Design review of the part built by this model. Coordinates are the model's own, in mm. A direction names the side the tool comes from. Round coordinates to 2 decimals unless told otherwise and drop trailing zeros. Loops run counter-clockwise (first coordinate to the right, second up) from the corner with the lowest first, then second, coordinate; pieces in that order, holes last. Notation, with made-up numbers: (-39, 60.25) - (4, 60.25) arc R20 ccw to (4, 66.25) - close; hole circle Ø3 at (-31.5, -8). An arc over 180 degrees is marked (long way). Use one line per item in the form item = value. Start each with the question number.
(1) We need section A-A, the plane z = 17. Write out the cut boundary in (x, y), then the cut area to 3 significant figures.
(2) Machinability: for faces 1 (the cylindrical face through (998.479, 10.525, -90.019)), 2 (the cylindrical face through (991.297, 90.986, 1.4)), which of the approach directions +Z, -Z, +X, -X, +Y, -Y give a long, thin tool a straight path to every point of the face, cutting with its end or side? Answer none if there is none.
(3) The part is to be moulded in two halves that separate along Y. For faces 3 (the cylindrical face through (1.479, 9.981, -89.475)), 4 (the cylindrical face through (2, 34, -52)), 5 (the flat face through (3, 39, 0)), say which applies: released by +Y, released by -Y, zero draft, split by the parting line, or undercut.
(4) Wall thickness on probe 1 along X at (y, z) = (57, -40.5); probe 2 along Y at (x, z) = (798.5, 64.5); probe 3 along X at (y, z) = (95.5, -28.5): over which ranges is each line inside the solid? List them lowest first. Write a range as [from, to].
(5) We need section B-B, the plane x = 613.5. Write out the cut boundary in (y, z), then the cut area to 3 significant figures.
(6) For pin 1 (1.5 mm diameter, centred on y = 89.5, z = -57, fed in from +X); pin 2 (8 mm diameter, centred on x = 395.5, z = 67.5, fed in from -Y), all flat-tipped, find the tip position at first contact; note any pin that passes through.
(7) We need section C-C, the plane z = 74.5. Write out the cut boundary in (x, y).
from build123d import *

# Parameters (mm, degrees)
BOSS_EXTRUDE1_DEPTH = 100
CUT_EXTRUDE1_DEPTH  = 1001
SKETCH4_R           = 10
CUT_EXTRUDE2_DEPTH  = 1001
FILLET3_R           = 35


with BuildPart() as part:
    # Sketch2 → Boss-Extrude1 (new body, symmetric)
    with BuildSketch(Plane.XY):
        with BuildLine():
            Line((0, 0), (0, 80))
            ThreePointArc((0, 80), (5.857864376, 94.142135624), (20, 100))
            Line((20, 100), (980, 100))
            ThreePointArc((980, 100), (994.142135624, 94.142135624), (1000, 80))
            Line((1000, 80), (1000, 0))
            Line((1000, 0), (997, 0))
            Line((997, 0), (997, 77))
            ThreePointArc((997, 77), (991.142135624, 91.142135624), (977, 97))
            Line((977, 97), (23, 97))
            ThreePointArc((23, 97), (8.857864376, 91.142135624), (3, 77))
            Line((3, 77), (3, 0))
            Line((3, 0), (0, 0))
        make_face()
    extrude(amount=BOSS_EXTRUDE1_DEPTH, both=True)

    # Sketch3 → Cut-Extrude1 (cut, through all)
    with BuildSketch(Plane(origin=(1000, 0, 0), x_dir=(0, 0, -1), z_dir=(1, 0, 0))):
        Polygon((-100, 0), (-50, 0), (-100, 80), align=None)
    extrude(amount=-CUT_EXTRUDE1_DEPTH, mode=Mode.SUBTRACT)

    # Sketch4 → Cut-Extrude2 (cut, through all)
    with BuildSketch(Plane(origin=(1000, 0, 0), x_dir=(0, 0, -1), z_dir=(1, 0, 0))):
        with Locations((60, 40)):
            Circle(SKETCH4_R)
    extrude(amount=-CUT_EXTRUDE2_DEPTH, mode=Mode.SUBTRACT)

    # Fillet3
    fillet3_edges = [part.edges().sort_by_distance(p)[0] for p in [
        (998.5, 0, -100),
        (1.5, 0, -100),
    ]]
    fillet(fillet3_edges, radius=FILLET3_R)


solid = part.part
Data:
q1.outline = (0, 0) - (3, 0) - (3, 77) arc R20 cw to (23, 97) - (977, 97) arc R20 cw to (997, 77) - (997, 0) - (1000, 0) - (1000, 80) arc R20 ccw to (980, 100) - (20, 100) arc R20 ccw to (0, 80) - close
q1.area = 3,580 mm^2
q2.face_1 = -Z, +X, -X, -Y
q2.face_2 = +Z, -Z, -Y
q3.face_3 = released by -Y
q3.face_4 = undercut
q3.face_5 = zero draft
q4.probe_1 = [0, 3], [997, 1000]
q4.probe_2 = [97, 100]
q4.probe_3 = [7.36, 15.4], [984.6, 992.64]
q5.outline = (97, -100) - (100, -100) - (100, 100) - (97, 100) - close
q5.area = 600 mm^2
q6.pin_1 = 997.98
q6.pin_2 = 97
q7.outline = (0, 39.2) - (3, 39.2) - (3, 77) arc R20 cw to (23, 97) - (977, 97) arc R20 cw to (997, 77) - (997, 39.2) - (1000, 39.2) - (1000, 80) arc R20 ccw to (980, 100) - (20, 100) arc R20 ccw to (0, 80) - close
